Could you check a few things on this model? Use its own coordinates, in mm. A direction names the side the tool comes from. Coordinates: 2 decimals unless noted, no trailing zeros. Order: outer loops, then holes, each group sorted by start corner. A loop starts at its lowest first (then second) coordinate and runs counter-clockwise, first axis right, second up. Notation, with made-up numbers: (60, 77.25) - (112, 77.25) arc R18 cw to (112, 86.25) - close; hole circle Ø11 at (23, -30.5). An arc over 180 degrees is marked (long way). One line per item, written item: value.
from build123d import *

# Parameters (mm, degrees)
F0_W         = 102.5
F0_H         = 20
F1_DEPTH     = 1
F2_W         = 102.5
F2_H         = 4.5
F3_DEPTH     = 1.5
F4_C1_SIZE2  = 0.45
F4_C1_SIZE   = 0.7794228634
F4_C2_SIZE2  = 0.7794228634
F4_C2_SIZE   = 0.45
F4_C3_SIZE2  = 0.7794228634
F4_C3_SIZE   = 0.45
F4_C4_SIZE2  = 0.7794228634
F4_C4_SIZE   = 0.45
F5_T1_DEPTH  = 2.4705771366
F5_T3_DEPTH  = 1
F5_T5_DEPTH  = 3.5
F5_T7_DEPTH  = 101.5
F5_T9_DEPTH  = 16.5365895505
F5_S13_W     = 0.51
F5_S13_H     = 0.51
F5_T14_DEPTH = 0.51
F5_S19_W     = 0.51
F5_S19_H     = 0.51
F5_T20_DEPTH = 0.51
F5_S25_W     = 0.51
F5_S25_H     = 0.51
F5_T26_DEPTH = 0.51
F5_S31_W     = 0.51
F5_S31_H     = 0.51
F5_T32_DEPTH = 0.51
F5_T39_DEPTH = 16.5365895505
F5_T43_DEPTH = 2.25
F5_T52_DEPTH = 16.5365895505
F5_T56_DEPTH = 2.25


# Not quite as in the source:
# - a fillet or chamfer that OpenCascade refuses, or shapes differently, is made with other operations: its cross-section is extruded or revolved along the edge and cut away or added


with BuildPart() as f1:
    # F0 (on Top) → F1 (new body)
    with BuildSketch(Plane.XY):
        with Locations((-51.25, 10)):
            Rectangle(F0_W, F0_H)
    extrude(amount=F1_DEPTH)

    # F2 (on face) → F3 (join)
    with BuildSketch(Plane.XY.offset(1)):
        with Locations((-51.25, 17.75)):
            Rectangle(F2_W, F2_H)
    extrude(amount=F3_DEPTH)

    # F4: chamfer of 0.45 x 0.7794228634 on 4 edges, made by hand

    # F4_c1
    f4_c1_edges = [f1.edges().sort_by_distance(p)[0] for p in [
        (-51.25, 0, 0),
    ]]
    f4_c1_side = f1.faces().sort_by_distance((-51.25, 0, 0.009))[0]
    chamfer(f4_c1_edges, length=F4_C1_SIZE, length2=F4_C1_SIZE2, reference=f4_c1_side)

    # F4_c2
    f4_c2_edges = [f1.edges().sort_by_distance(p)[0] for p in [
        (-51.25, 20, 0),
    ]]
    f4_c2_side = f1.faces().sort_by_distance((-51.25, 19.991, 0))[0]
    chamfer(f4_c2_edges, length=F4_C2_SIZE, length2=F4_C2_SIZE2, reference=f4_c2_side)

    # F4_c3
    f4_c3_edges = [f1.edges().sort_by_distance(p)[0] for p in [
        (0, 10, 0),
    ]]
    f4_c3_side = f1.faces().sort_by_distance((-0.009, 10, 0))[0]
    chamfer(f4_c3_edges, length=F4_C3_SIZE, length2=F4_C3_SIZE2, reference=f4_c3_side)

    # F4_c4
    f4_c4_edges = [f1.edges().sort_by_distance(p)[0] for p in [
        (-102.5, 10, 0),
    ]]
    f4_c4_side = f1.faces().sort_by_distance((-102.491, 10, 0))[0]
    chamfer(f4_c4_edges, length=F4_C4_SIZE, length2=F4_C4_SIZE2, reference=f4_c4_side)

    # F5: fillet of radius 0.5 on 10 edges, made by hand

    # F5_s2 → F5_t1 (cut)
    with BuildSketch(Plane.XY.offset(-0.4705771366)):
        with BuildLine():
            ThreePointArc((-102, 20), (-102.3535533906, 19.8535533906), (-102.5, 19.5))
            Line((-102.5, 19.5), (-102.5, 20))
            Line((-102.5, 20), (-102, 20))
        make_face()
        with BuildLine():
            ThreePointArc((-0.5, 20), (-0.1464466094, 19.8535533906), (0, 19.5))
            Line((0, 19.5), (0, 20))
            Line((0, 20), (-0.5, 20))
        make_face()
    extrude(amount=F5_T1_DEPTH, mode=Mode.SUBTRACT)

    # F5_s4 → F5_t3 (cut)
    with BuildSketch(Plane.XY.offset(1)):
        with BuildLine():
            ThreePointArc((-102.5, 16), (-102.3535533906, 15.6464466094), (-102, 15.5))
            Line((-102, 15.5), (-102.5, 15.5))
            Line((-102.5, 15.5), (-102.5, 16))
        make_face()
        with BuildLine():
            ThreePointArc((0, 16), (-0.1464466094, 15.6464466094), (-0.5, 15.5))
            Line((-0.5, 15.5), (0, 15.5))
            Line((0, 15.5), (0, 16))
        make_face()
    extrude(amount=F5_T3_DEPTH, mode=Mode.SUBTRACT)

    # F5_s6 → F5_t5 (cut)
    with BuildSketch(Plane.XZ.offset(-19.5)):
        with BuildLine():
            ThreePointArc((-102.5, 2), (-102.3535533906, 2.3535533906), (-102, 2.5))
            Line((-102, 2.5), (-102.5, 2.5))
            Line((-102.5, 2.5), (-102.5, 2))
        make_face()
        with BuildLine():
            ThreePointArc((0, 2), (-0.1464466094, 2.3535533906), (-0.5, 2.5))
            Line((-0.5, 2.5), (0, 2.5))
            Line((0, 2.5), (0, 2))
        make_face()
    extrude(amount=F5_T5_DEPTH, mode=Mode.SUBTRACT)

    # F5_s8 → F5_t7 (cut)
    with BuildSketch(Plane.YZ.offset(-102)):
        with BuildLine():
            ThreePointArc((20, 2), (19.8535533906, 2.3535533906), (19.5, 2.5))
            Line((19.5, 2.5), (20, 2.5))
            Line((20, 2.5), (20, 2))
        make_face()
        with BuildLine():
            ThreePointArc((16, 2.5), (15.6464466094, 2.3535533906), (15.5, 2))
            Line((15.5, 2), (15.5, 2.5))
            Line((15.5, 2.5), (16, 2.5))
        make_face()
    extrude(amount=F5_T7_DEPTH, mode=Mode.SUBTRACT)

    # F5_s10 → F5_t9 (cut)
    with BuildSketch(Plane.XZ.offset(-15.5)):
        with BuildLine():
            ThreePointArc((-102.5, 0.7794228634), (-102.3201923811, 0.9414246435), (-102.0853641798, 1))
            Line((-102.0853641798, 1), (-102.5, 1))
            Line((-102.5, 1), (-102.5, 0.7794228634))
        make_face()
        with BuildLine():
            ThreePointArc((0, 0.7794228634), (-0.1798076189, 0.9414246435), (-0.4146358202, 1))
            Line((-0.4146358202, 1), (0, 1))
            Line((0, 1), (0, 0.7794228634))
        make_face()
    extrude(amount=F5_T9_DEPTH, mode=Mode.SUBTRACT)


with BuildPart() as f5_tool12:
    # F5_s13 → F5_t14 (new body)
    with BuildSketch(Plane.XY.offset(2)):
        with Locations((-102.255, 19.755)):
            Rectangle(F5_S13_W, F5_S13_H)
    extrude(amount=F5_T14_DEPTH)

    # F5_s15 → F5_t16 (revolve, cut)
    with BuildSketch(Plane(origin=(-102, 19.5, 2), x_dir=(0.7071067812, -0.7071067812, 0), z_dir=(-0.7071067812, -0.7071067812, 0))):
        with BuildLine():
            ThreePointArc((0, -0.5), (0.5, 0), (0, 0.5))
            Line((0, 0.5), (0, -0.5))
        make_face()
    revolve(axis=Axis((-102, 19.5, 2), (0, 0, 1)), mode=Mode.SUBTRACT)


with BuildPart() as f1_1:
    add(f1.part)

    # F5_t11: cut F5_tool12
    add(f5_tool12.part, mode=Mode.SUBTRACT)


with BuildPart() as f5_tool18:
    # F5_s19 → F5_t20 (new body)
    with BuildSketch(Plane.XY.offset(2)):
        with Locations((-102.255, 15.745)):
            Rectangle(F5_S19_W, F5_S19_H)
    extrude(amount=F5_T20_DEPTH)

    # F5_s21 → F5_t22 (revolve, cut)
    with BuildSketch(Plane(origin=(-102, 16, 2), x_dir=(0.7071067812, 0.7071067812, 0), z_dir=(0.7071067812, -0.7071067812, 0))):
        with BuildLine():
            ThreePointArc((0, -0.5), (0.5, 0), (0, 0.5))
            Line((0, 0.5), (0, -0.5))
        make_face()
    revolve(axis=Axis((-102, 16, 2), (0, 0, 1)), mode=Mode.SUBTRACT)


with BuildPart() as f1_2:
    add(f1_1.part)

    # F5_t17: cut F5_tool18
    add(f5_tool18.part, mode=Mode.SUBTRACT)


with BuildPart() as f5_tool24:
    # F5_s25 → F5_t26 (new body)
    with BuildSketch(Plane.XY.offset(2)):
        with Locations((-0.245, 19.755)):
            Rectangle(F5_S25_W, F5_S25_H)
    extrude(amount=F5_T26_DEPTH)

    # F5_s27 → F5_t28 (revolve, cut)
    with BuildSketch(Plane(origin=(-0.5, 19.5, 2), x_dir=(-0.7071067812, -0.7071067812, 0), z_dir=(-0.7071067812, 0.7071067812, 0))):
        with BuildLine():
            ThreePointArc((0, -0.5), (0.5, 0), (0, 0.5))
            Line((0, 0.5), (0, -0.5))
        make_face()
    revolve(axis=Axis((-0.5, 19.5, 2), (0, 0, 1)), mode=Mode.SUBTRACT)


with BuildPart() as f1_3:
    add(f1_2.part)

    # F5_t23: cut F5_tool24
    add(f5_tool24.part, mode=Mode.SUBTRACT)


with BuildPart() as f5_tool30:
    # F5_s31 → F5_t32 (new body)
    with BuildSketch(Plane.XY.offset(2)):
        with Locations((-0.245, 15.745)):
            Rectangle(F5_S31_W, F5_S31_H)
    extrude(amount=F5_T32_DEPTH)

    # F5_s33 → F5_t34 (revolve, cut)
    with BuildSketch(Plane(origin=(-0.5, 16, 2), x_dir=(-0.7071067812, 0.7071067812, 0), z_dir=(0.7071067812, 0.7071067812, 0))):
        with BuildLine():
            ThreePointArc((0, -0.5), (0.5, 0), (0, 0.5))
            Line((0, 0.5), (0, -0.5))
        make_face()
    revolve(axis=Axis((-0.5, 16, 2), (0, 0, 1)), mode=Mode.SUBTRACT)


with BuildPart() as f1_4:
    add(f1_3.part)

    # F5_t29: cut F5_tool30
    add(f5_tool30.part, mode=Mode.SUBTRACT)


with BuildPart() as f5_tool37:
    # F5_s38 → F5_t39 (new body)
    with BuildSketch(Plane.XZ.offset(-16.5365895505)):
        with BuildLine():
            ThreePointArc((-102.5, 0.7794228634), (-102.3201923811, 0.9414246435), (-102.0853641798, 1))
            Line((-102.0853641798, 1), (-102.5, 1))
            Line((-102.5, 1), (-102.5, 0.7794228634))
        make_face()
    extrude(amount=F5_T39_DEPTH)

    split(bisect_by=Plane.XZ.offset(-15.5), keep=Keep.BOTTOM)


with BuildPart() as f5_tool41:
    # F5_s42 → F5_t43 (new body)
    with BuildSketch(Plane.XY.offset(-0.25)):
        with BuildLine():
            ThreePointArc((-102.5, 16), (-102.3535533906, 15.6464466094), (-102, 15.5))
            Line((-102, 15.5), (-102.5, 15.5))
            Line((-102.5, 15.5), (-102.5, 16))
        make_face()
    extrude(amount=F5_T43_DEPTH)

    split(bisect_by=Plane.XY, keep=Keep.TOP)

    split(bisect_by=Plane(origin=(-76.5375, 0, -44.1889462281), x_dir=(0, 1, 0), z_dir=(0.8660254038, 0, 0.5)), keep=Keep.TOP)

    split(bisect_by=Plane.XY.offset(1), keep=Keep.BOTTOM)


with BuildPart() as f5_tool37_1:
    add(f5_tool37.part)

    # F5_t47: intersect F5_tool41
    add(f5_tool41.part, mode=Mode.INTERSECT)


with BuildPart() as f1_5:
    add(f1_4.part)

    # F5_t35: cut F5_tool37
    add(f5_tool37_1.part, mode=Mode.SUBTRACT)


with BuildPart() as f5_tool50:
    # F5_s51 → F5_t52 (new body)
    with BuildSketch(Plane.XZ):
        with BuildLine():
            ThreePointArc((0, 0.7794228634), (-0.1798076189, 0.9414246435), (-0.4146358202, 1))
            Line((-0.4146358202, 1), (0, 1))
            Line((0, 1), (0, 0.7794228634))
        make_face()
    extrude(amount=-F5_T52_DEPTH)

    split(bisect_by=Plane.XZ.offset(-15.5), keep=Keep.BOTTOM)


with BuildPart() as f5_tool54:
    # F5_s55 → F5_t56 (new body)
    with BuildSketch(Plane.XY.offset(-0.25)):
        with BuildLine():
            ThreePointArc((0, 16), (-0.1464466094, 15.6464466094), (-0.5, 15.5))
            Line((-0.5, 15.5), (0, 15.5))
            Line((0, 15.5), (0, 16))
        make_face()
    extrude(amount=F5_T56_DEPTH)

    split(bisect_by=Plane.XY, keep=Keep.TOP)

    split(bisect_by=Plane(origin=(-0.3375, 0, 0.1948557159), x_dir=(0, 1, 0), z_dir=(-0.8660254038, 0, 0.5)), keep=Keep.TOP)

    split(bisect_by=Plane.XY.offset(1), keep=Keep.BOTTOM)


with BuildPart() as f5_tool50_1:
    add(f5_tool50.part)

    # F5_t60: intersect F5_tool54
    add(f5_tool54.part, mode=Mode.INTERSECT)


with BuildPart() as f1_6:
    add(f1_5.part)

    # F5_t48: cut F5_tool50
    add(f5_tool50_1.part, mode=Mode.SUBTRACT)


solid = f1_6.part
Item 1: I want a section at A-A on z = 1.4. Please give me the cut outline in (x, y).
Conclusion:
outline: (-102.5, 16) arc R0.5 ccw to (-102, 15.5) - (-0.5, 15.5) arc R0.5 ccw to (0, 16) - (0, 19.5) arc R0.5 ccw to (-0.5, 20) - (-102, 20) arc R0.5 ccw to (-102.5, 19.5) - close
Item 2: I'm going to push flat-ended pins straight in: pin 1 Ø0.5 at (x, z) = (-54.5, 1.5) entering from -Y; pin 2 Ø8 at (x, y) = (-55.5, 10.5) entering from +Z. Where does each tip first touch, or does it pass through?
Conclusion:
pin 1: y = 15.5
pin 2: z = 1
Item 3: If I drill on probe 1 along X at (y, z) = (6.25, 0.5); probe 2 along Z at (x, y) = (-44.5, 3.25); probe 3 along Y at (x, z) = (-60, 2.1), over which ranges is the centre line in solid material (lowest first)?
Conclusion:
probe 1: -102.34 to -0.16
probe 2: 0 to 1
probe 3: 15.51 to 19.99
Item 4: I want a section at C-C on y = 13. Please give me the cut outline in (x, z).
Conclusion:
outline: (-102.5, 0.78) - (-102.05, 0) - (-0.45, 0) - (0, 0.78) arc R0.5 ccw to (-0.41, 1) - (-102.09, 1) arc R0.5 ccw to start
Item 5: For faces 1 (the face through (-52, 10, 0)), 2 (the face through (-51, 8, 1)), which set-ups out of +Z, -Z, +X, -X, +Y, -Y let a thin tool reach every point of the face, with its end or its side?
Conclusion:
face 1: -Z, +X, -X, +Y, -Y
face 2: +Z, +X, -X, -Y
Item 6: I want a section at B-B on x = -10. Please give me the cut outline in (y, z), then the cut area to 3 significant figures.
Conclusion:
outline: (0, 0.78) - (0.45, 0) - (19.55, 0) - (20, 0.78) - (20, 2) arc R0.5 ccw to (19.5, 2.5) - (16, 2.5) arc R0.5 ccw to (15.5, 2) - (15.5, 1) - (0, 1) - close
area: 26.3 mm²
